Can you work these out from the model? Positions are in its coordinate system, mm. A direction names the side the tool comes from. Give positions to 0.01 mm unless a question says otherwise; leave off trailing zeros. Order: outer loops, then holes, each group sorted by start corner. A loop starts at its lowest first (then second) coordinate and runs counter-clockwise, first axis right, second up. Notation, with made-up numbers: M 37.5,5 L 44.5,5 A9 cw 44.5,17 Z; hole C 57.5,36 d7. An arc over 180 degrees is marked long. Write each question's results on one line, items separated by ' | '.
from build123d import *

# Parameters (mm, degrees)
BOSS_EXTRUDE1_START             = 170.258318
SKETCH6_R                       = 14.2875
BOSS_EXTRUDE1_DEPTH             = 6.35
F_5_0MM_DOWEL_HOLE1_D           = 5
F_5_0MM_DOWEL_HOLE1_DEPTH       = 25.4
F_5_0MM_DOWEL_HOLE1_CSINK_D     = 5.05
F_5_0MM_DOWEL_HOLE1_CSINK_ANGLE = 90
F_5_0MM_DOWEL_HOLE1_TIP         = 1.502151548


with BuildPart() as part:
    # Sketch6 → Boss-Extrude1 (new body)
    with BuildSketch(Plane(origin=(0, 0, 0), x_dir=(0, 0, -1), z_dir=(1, 0, 0)).offset(BOSS_EXTRUDE1_START)):
        Polygon((74.6125, 36.5633), (128.5875, 36.5633), (128.5875, 96.52), (114.3, 96.52), (114.3, 76.2), (88.9, 76.2), (88.9, 96.52), (74.6125, 96.52), align=None)
        with Locations((101.6, 54.0258)):
            Circle(SKETCH6_R, mode=Mode.SUBTRACT)
    extrude(amount=-BOSS_EXTRUDE1_DEPTH)

    # Ø5.0mm Dowel Hole1
    with Locations(Plane(origin=(0, 96.52, 0), x_dir=(1, 0, 0), z_dir=(0, 1, 0))):
        with Locations((167.083317581, 122.2375), (167.083317581, 80.9625)):
            CounterSinkHole(F_5_0MM_DOWEL_HOLE1_D / 2, F_5_0MM_DOWEL_HOLE1_CSINK_D / 2, depth=F_5_0MM_DOWEL_HOLE1_DEPTH, counter_sink_angle=F_5_0MM_DOWEL_HOLE1_CSINK_ANGLE)
            with Locations((0, 0, -(F_5_0MM_DOWEL_HOLE1_DEPTH + F_5_0MM_DOWEL_HOLE1_TIP / 2))):  # 118° drill point
                Cone(0, F_5_0MM_DOWEL_HOLE1_D / 2, F_5_0MM_DOWEL_HOLE1_TIP, mode=Mode.SUBTRACT)


solid = part.part
(1) Imagine slicing it at A-A, the plane y = 83. Write out the boundary of the cut face in (x, z), plus the area to 3 significant figures.
Data:
outline: M 163.91,-128.59 L 170.26,-128.59 L 170.26,-114.3 L 163.91,-114.3 Z; M 163.91,-88.9 L 170.26,-88.9 L 170.26,-74.61 L 163.91,-74.61 Z; hole C 167.08,-122.24 d5; hole C 167.08,-80.96 d5 | area: 142 mm2
(2) Imagine slicing it at B-B, the plane z = -101.6. Write out the boundary of the cut face in (x, y).
Data:
outline: M 163.91,36.56 L 170.26,36.56 L 170.26,39.74 L 163.91,39.74 Z; M 163.91,68.31 L 170.26,68.31 L 170.26,76.2 L 163.91,76.2 Z
(3) I need wall thicknesses on L1, parallel to Z at x = 167, y = 91; L2, parallel to X at y = 86, z = -81; L3, parallel to Z at x = 168.75, y = 90.5. Which ranges of each line are inside material? Lowest first, please. Write a range as from..to.
Data:
L1: z = -128.59..-124.74, -119.74..-114.3, -88.9..-83.46, -78.46..-74.61 | L2: x = 163.91..164.58, 169.58..170.26 | L3: z = -128.59..-124.1, -120.37..-114.3, -88.9..-82.83, -79.1..-74.61
(4) For faces 1 (the face through (169, 96.52, -120)), 2 (the face through (167, 76.2, -102)), 3 (the face through (169.067, 83.63, -79.441)), which set-ups out of +Z, -Z, +X, -X, +Y, -Y let a thin tool reach every point of the face, with its end or its side?
Data:
face 1: +Z, -Z, +X, -X, +Y | face 2: +X, -X, +Y | face 3: +Y
(5) We'd pull the mould along Z, two halves only. Please class faces 4 (the face through (167.128, 45.332, -90.262)), 5 (the face through (167, 66, -128.588)), 6 (the face through (170.258, 67, -95)): +Z half, -Z half, draft (parallel to the pull), parting line (faces both ways), or undercut.
Data:
face 4: undercut | face 5: -Z half | face 6: draft
(6) Will this pin go through, and if not, where does the flat tip stop? P1, Ø3, axis at x = 166, z = -90.5, coming from the +Y side.
Data:
P1: stops at y = 76.2
(7) Imagine slicing it at C-C, the plane y = 46.5. Write out the boundary of the cut face in (x, z), plus the area to 3 significant figures.
Data:
outline: M 163.91,-128.59 L 170.26,-128.59 L 170.26,-113.74 L 163.91,-113.74 Z; M 163.91,-89.46 L 170.26,-89.46 L 170.26,-74.61 L 163.91,-74.61 Z | area: 189 mm2
